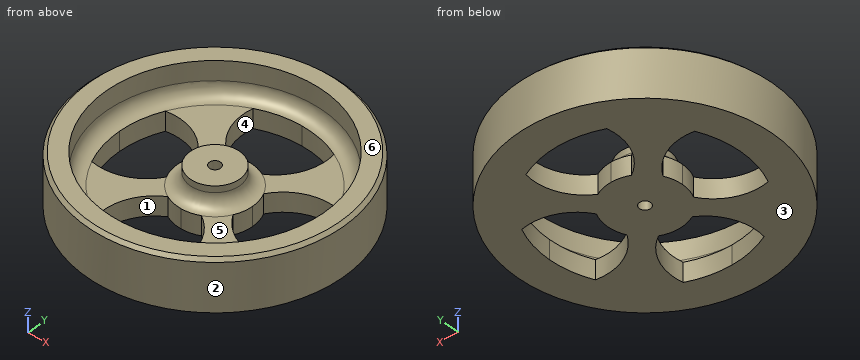
```python
from build123d import *

# Parameters (mm, degrees)
F2_SIZE  = 0.5
F4_DEPTH = 3


with BuildPart() as f1:
    # F0 (on Front) → F1 (revolve)
    with BuildSketch(Plane.XZ):
        with BuildLine():
            Line((0.8636, 6), (0.8636, 0))
            Line((0.8636, 0), (20, 0))
            Line((20, 0), (20, 8))
            Line((20, 8), (17, 8))
            Line((17, 8), (17, 5))
            ThreePointArc((17, 5), (16.4142135624, 3.5857864376), (15, 3))
            Line((15, 3), (5.8636, 3))
            ThreePointArc((5.8636, 3), (4.4493864376, 3.5857864376), (3.8636, 5))
            Line((3.8636, 5), (3.8636, 6))
            Line((3.8636, 6), (0.8636, 6))
        make_face()
    revolve(axis=Axis((0, 0, 9.2181318827), (0, 0, 1)))

    # F2
    f2_edges = [f1.edges().sort_by_distance(p)[0] for p in [
        (-20, 0, 8),
    ]]
    chamfer(f2_edges, length=F2_SIZE)

    # F3 (on face) → F4 (cut, through all)
    with BuildSketch(Plane.XY.offset(3)):
        with BuildLine():
            ThreePointArc((13.5867362981, 6.3561463771), (8.8277844457, 5.8106888065), (5.2335374725, 2.6442183124))
            ThreePointArc((5.2335374725, 2.6442183124), (5.7039098557, 1.3591237317), (5.8636, 0))
            ThreePointArc((5.8636, 0), (5.7039098557, -1.3591237317), (5.2335374725, -2.6442183124))
            ThreePointArc((5.2335374725, -2.6442183124), (8.8277844457, -5.8106888065), (13.5867362981, -6.3561463771))
            ThreePointArc((13.5867362981, -6.3561463771), (14.6424220071, -3.2556839166), (15, 0))
            ThreePointArc((15, 0), (14.6424220071, 3.2556839166), (13.5867362981, 6.3561463771))
        make_face()
        with BuildLine():
            ThreePointArc((0, 15), (-3.2556839166, 14.6424220071), (-6.3561463771, 13.5867362981))
            ThreePointArc((-6.3561463771, 13.5867362981), (-5.8106888065, 8.8277844457), (-2.6442183124, 5.2335374725))
            ThreePointArc((-2.6442183124, 5.2335374725), (-1.3591237317, 5.7039098557), (0, 5.8636))
            ThreePointArc((0, 5.8636), (1.3591237317, 5.7039098557), (2.6442183124, 5.2335374725))
            ThreePointArc((2.6442183124, 5.2335374725), (5.8106888065, 8.8277844457), (6.3561463771, 13.5867362981))
            ThreePointArc((6.3561463771, 13.5867362981), (3.2556839166, 14.6424220071), (0, 15))
        make_face()
        with BuildLine():
            ThreePointArc((-15, 0), (-14.6424220071, -3.2556839166), (-13.5867362981, -6.3561463771))
            ThreePointArc((-13.5867362981, -6.3561463771), (-8.8277844457, -5.8106888065), (-5.2335374725, -2.6442183124))
            ThreePointArc((-5.2335374725, -2.6442183124), (-5.7039098557, -1.3591237317), (-5.8636, 0))
            ThreePointArc((-5.8636, 0), (-5.7039098557, 1.3591237317), (-5.2335374725, 2.6442183124))
            ThreePointArc((-5.2335374725, 2.6442183124), (-8.8277844457, 5.8106888065), (-13.5867362981, 6.3561463771))
            ThreePointArc((-13.5867362981, 6.3561463771), (-14.6424220071, 3.2556839166), (-15, 0))
        make_face()
        with BuildLine():
            ThreePointArc((0, -15), (3.2556839166, -14.6424220071), (6.3561463771, -13.5867362981))
            ThreePointArc((6.3561463771, -13.5867362981), (5.8106888065, -8.8277844457), (2.6442183124, -5.2335374725))
            ThreePointArc((2.6442183124, -5.2335374725), (1.3591237317, -5.7039098557), (0, -5.8636))
            ThreePointArc((0, -5.8636), (-1.3591237317, -5.7039098557), (-2.6442183124, -5.2335374725))
            ThreePointArc((-2.6442183124, -5.2335374725), (-5.8106888065, -8.8277844457), (-6.3561463771, -13.5867362981))
            ThreePointArc((-6.3561463771, -13.5867362981), (-3.2556839166, -14.6424220071), (0, -15))
        make_face()
    extrude(amount=-F4_DEPTH, mode=Mode.SUBTRACT)


solid = f1.part
```
Read the model definition and answer for the solid it produces. Units are mm, in the model's axes. Face numbers are marked on the shaded views. A direction names the side the tool comes from. Give positions to 0.01 mm unless a question says otherwise; leave off trailing zeros. Write each loop counter-clockwise with the first axis right and the second up, starting at its lowest first coordinate (ties: lowest second). Pieces come first, ordered by that corner, then holes. Notation, with made-up numbers: (-35, 9) -> (-9, 9) arc R9 cw to (-9, 19) -> close; hole circle Ø5 at (-6.5, 44). An arc over 180 degrees is marked (long way). Answer in a Markdown table with one row per item.
1) Each of these flat-tipped pins is pushed along its axis until it touches: pin 1 Ø9 at (x, y) = (7, -7.5) entering from +Z; pin 2 Ø1.5 at (x, z) = (12, 2.5) entering from +Y; pin 3 Ø4 at (x, y) = (1.5, 1) entering from +Z. Where does it stop, or does it pass through?
Results list:
| item | result |
|---|---|
| pin 1 | z = 3 |
| pin 2 | y = 16.54 |
| pin 3 | z = 6 |
2) Straight lines are drawn through the part: line 1 (Y direction, x = 5, z = 0.75); line 2 (X direction, y = 2.5, z = 4.5); line 3 (Y direction, x = 0, z = 7.35). For each, find the intervals that lie inside material, in ascending order. Write a range as [from, to].
Results list:
| item | result |
|---|---|
| line 1 | [-19.36, -14.14], [-7.41, 7.41], [14.14, 19.36] |
| line 2 | [-19.84, -16.75], [-3.03, 3.03], [16.75, 19.84] |
| line 3 | [-20, -17], [17, 20] |
3) Determine the mould class of the marked faces 1, 2 and 3 for opening direction X: released by +X, released by -X, zero draft, split by the parting line, or undercut.
Results list:
| item | result |
|---|---|
| face 1 | undercut |
| face 2 | split by the parting line |
| face 3 | zero draft |
4) A tool of negligible diameter and unlimited length cuts with its end or side. For the marked faces 4, 5 and 6, from which of +Z, -Z, +X, -X, +Y, -Y can it reach the whole face along a straight path? Write none if from no direction.
Results list:
| item | result |
|---|---|
| face 4 | +Z, -Z |
| face 5 | +Z |
| face 6 | +Z, +X, -X, +Y, -Y |
5) Section A-A on z = 2 is taken. Give the vertices of the cut face in (x, y), plus the area to 3 significant figures.
Results list:
| item | result |
|---|---|
| outline | circle Ø40 at (0, 0); hole (-13.59, -6.36) arc R8 ccw to (-5.23, -2.64) arc R5.86 cw to (-5.23, 2.64) arc R8 ccw to (-13.59, 6.36) arc R15 ccw to start; hole (-6.36, -13.59) arc R15 ccw to (6.36, -13.59) arc R8 ccw to (2.64, -5.23) arc R5.86 cw to (-2.64, -5.23) arc R8 ccw to start; hole (-6.36, 13.59) arc R8 ccw to (-2.64, 5.23) arc R5.86 cw to (2.64, 5.23) arc R8 ccw to (6.36, 13.59) arc R15 ccw to start; hole circle Ø1.73 at (0, 0); hole (5.23, -2.64) arc R8 ccw to (13.59, -6.36) arc R15 ccw to (13.59, 6.36) arc R8 ccw to (5.23, 2.64) arc R5.86 cw to start |
| area | 843 mm^2 |
